Part print with two shaded views. Sizes in mm from the minimum x, y, z corner. A direction names the side the tool comes from. Give positions to 0.01 mm unless a question says otherwise; leave off trailing zeros. Order: outer loops, then holes, each group sorted by start corner. A loop starts at its lowest first (then second) coordinate and runs counter-clockwise, first axis right, second up. Notation, with made-up numbers: (-4, -39) -> (7, -39) arc R18 ccw to (7, -24) -> close; hole circle Ø11 at (34, 55.25). An arc over 180 degrees is marked (long way). Answer in a Markdown table with one row per item. Add a question column.
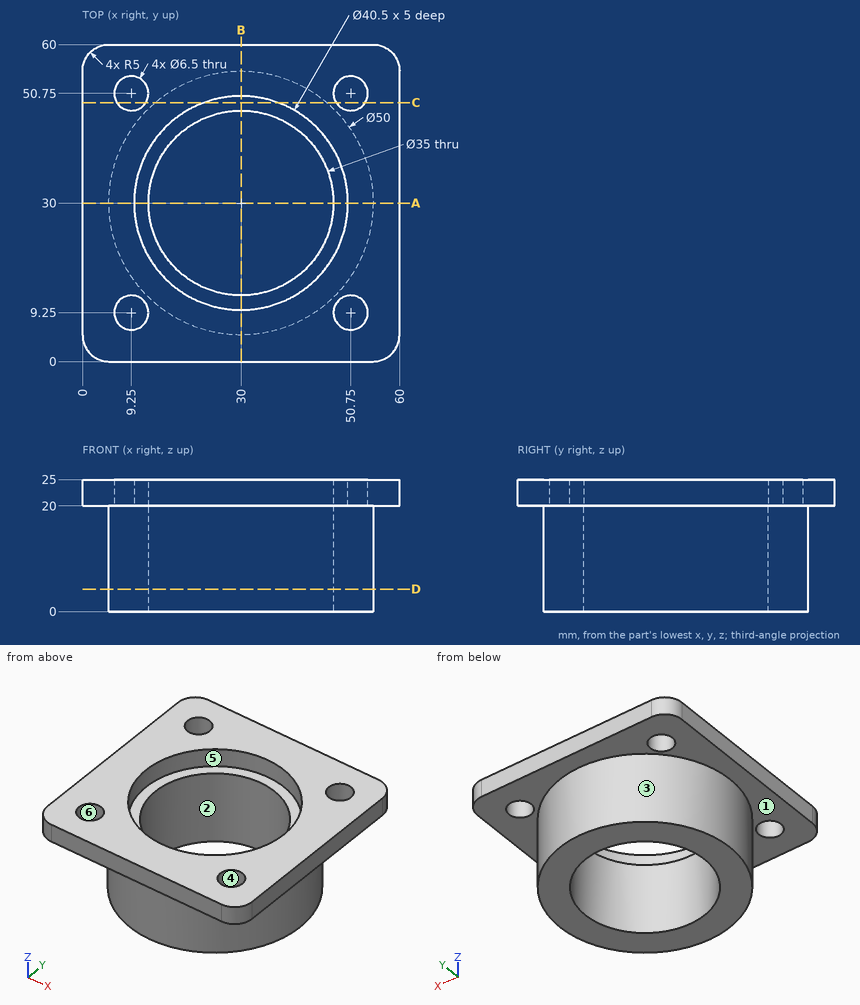
Item 1: Saw through at A-A on y = 30. List the corners of the cut face in (x, z).
Item 2: Two-plate mould, pull along Y, no slides. Class the marked faces 1, 2, 3 and 4: pulls with the +Y half, pulls with the -Y half, needs draft (parallel to the pull), parting line crosses it, or undercut.
Item 3: Saw through at C-C on y = 49. List the corners of the cut face in (x, z), plus the area to 3 significant figures.
Item 4: Saw through at D-D on z = 4.25. List the corners of the cut face in (x, y).
Item 5: Wall check: line 1 (Y direction, x = 50.75, z = 21.2); line 2 (X direction, y = 29.5, z = 13) (3 decimals); line 3 (Y direction, x = 30, z = 21.6). Give the ranges that are in metal, low to high.
Item 6: Which spindle directions (+Z, -Z, +X, -X, +Y, -Y) get a long thin tool onto all of the face, cutting with end or side? Do the marked faces 5 and 6. Say none if no direction does.
Item 7: Pin check, flat tips, straight feed: pin 1 Ø12 at (y, z) = (40, 4) entering from +X; pin 2 Ø4 at (x, y) = (9.25, 50.75) entering from -Z; pin 3 Ø1.5 at (x, z) = (39.5, 7) entering from +Y; pin 4 Ø2 at (y, z) = (9.5, 9) entering from -X. Stop position of each tip, or through.
Evaluation:
| question | item | result |
|---|---|---|
| 1 | outline | (0, 20) -> (5, 20) -> (5, 0) -> (12.5, 0) -> (12.5, 20) -> (9.75, 20) -> (9.75, 25) -> (0, 25) -> close; (47.5, 0) -> (55, 0) -> (55, 20) -> (60, 20) -> (60, 25) -> (50.25, 25) -> (50.25, 20) -> (47.5, 20) -> close |
| 2 | face 1 | needs draft |
| 2 | face 2 | undercut |
| 2 | face 3 | parting line crosses it |
| 2 | face 4 | undercut |
| 3 | outline | (0, 20) -> (6.51, 20) -> (6.51, 25) -> (0, 25) -> close; (11.99, 20) -> (13.75, 20) -> (13.75, 0) -> (46.25, 0) -> (46.25, 20) -> (48.01, 20) -> (48.01, 25) -> (37, 25) -> (37, 20) -> (23, 20) -> (23, 25) -> (11.99, 25) -> close; (53.49, 20) -> (60, 20) -> (60, 25) -> (53.49, 25) -> close |
| 3 | area | 825 mm2 |
| 4 | outline | circle Ø50 at (30, 30); hole circle Ø35 at (30, 30) |
| 5 | line 1 | y = 0 to 6, 12.5 to 47.5, 54 to 60 |
| 5 | line 2 | x = 5.005 to 12.507, 47.493 to 54.995 |
| 5 | line 3 | y = 0 to 9.75, 50.25 to 60 |
| 6 | face 5 | +Z |
| 6 | face 6 | +Z, -Z |
| 7 | pin 1 | stops at x = 54.68 |
| 7 | pin 2 | passes through |
| 7 | pin 3 | stops at y = 53.42 |
| 7 | pin 4 | stops at x = 14.36 |
